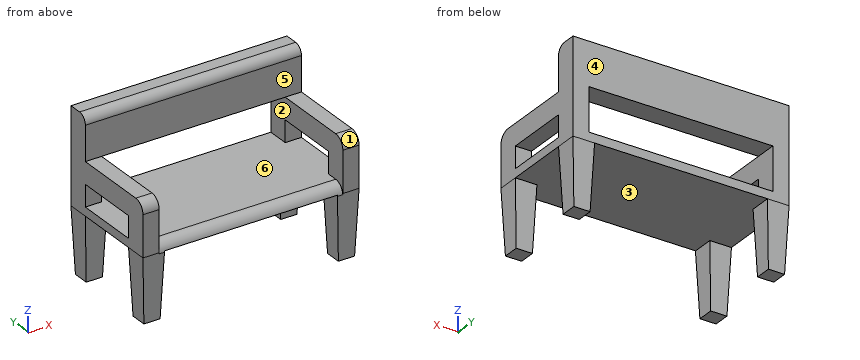
```python
from build123d import *

# Parameters (mm, degrees)
F0_W         = 200
F0_H         = 100
F1_DEPTH     = 8
F2_W         = 20
F2_H         = 20
F4_W         = 15
F4_H         = 15
F8_W         = 15
F8_H         = 20
F9_DEPTH     = 80
F11_W        = 20
F11_H        = 40
F12_DEPTH    = 170
F14_DEPTH    = 80
F15_W        = 15
F15_H        = 20
F16_DEPTH    = 20
F18_R        = 10
F19_R        = 10
F20_T1_DEPTH = 170
F21_R        = 8


# Not quite as in the source:
# - a fillet or chamfer that OpenCascade refuses, or shapes differently, is made with other operations: its cross-section is extruded or revolved along the edge and cut away or added


with BuildPart() as f1:
    # F0 (on Top) → F1 (new body)
    with BuildSketch(Plane.XY):
        Rectangle(F0_W, F0_H)
    extrude(amount=F1_DEPTH)

    # F2 (on face) → F5 section 0
    with BuildSketch(Plane(origin=(0, 0, 0), x_dir=(1, 0, 0), z_dir=(0, 0, -1))):
        with Locations((-90, 40)):
            Rectangle(F2_W, F2_H)
    # F4 (on offset) → F5 section 1
    with BuildSketch(Plane.XY.offset(-60)):
        with Locations((-90, -40)):
            Rectangle(F4_W, F4_H)
    loft()

    # F6: F1 across plane


with BuildPart() as f1_1:
    add(f1.part)
    add(f1.part.mirror(Plane.XZ))

    # F7: F1 across plane


with BuildPart() as f1_2:
    add(f1_1.part)
    add(f1_1.part.mirror(Plane.YZ))

    # F8 (on face) → F9 (join)
    with BuildSketch(Plane.XY.offset(8)):
        with Locations((-92.5, 40)):
            Rectangle(F8_W, F8_H)
    extrude(amount=F9_DEPTH)

    # F10: F1 across plane


with BuildPart() as f1_3:
    add(f1_2.part)
    add(f1_2.part.mirror(Plane.YZ))

    # F11 (on face) → F12 (join)
    with BuildSketch(Plane.YZ.offset(-85)):
        with Locations((40, 68)):
            Rectangle(F11_W, F11_H)
    extrude(amount=F12_DEPTH)

    # F13 (on face) → F14 (join)
    with BuildSketch(Plane.XZ.offset(-30)):
        Polygon((-85, 28), (-85, 48), (-92.5, 48), (-100, 48), (-100, 28), align=None)
    extrude(amount=F14_DEPTH)

    # F15 (on face) → F16 (join)
    with BuildSketch(Plane(origin=(0, 0, 28), x_dir=(1, 0, 0), z_dir=(0, 0, -1))):
        with Locations((-92.5, 40)):
            Rectangle(F15_W, F15_H)
    extrude(amount=F16_DEPTH)

    # F17: F1 across plane


with BuildPart() as f1_4:
    add(f1_3.part)
    add(f1_3.part.mirror(Plane.YZ))

    # F18
    f18_edges = [f1_4.edges().sort_by_distance(p)[0] for p in [
        (92.5, -50, 48),
    ]]
    fillet(f18_edges, radius=F18_R)

    # F19
    f19_edges = [f1_4.edges().sort_by_distance(p)[0] for p in [
        (-92.5, -50, 48),
    ]]
    fillet(f19_edges, radius=F19_R)

    # F20: fillet of radius 10 on 1 edges, made by hand

    # F20_s2 → F20_t1 (cut)
    with BuildSketch(Plane.YZ.offset(-85)):
        with BuildLine():
            ThreePointArc((-50, -2), (-47.0710678119, 5.0710678119), (-40, 8))
            Line((-40, 8), (-50, 8))
            Line((-50, 8), (-50, -2))
        make_face()
    extrude(amount=F20_T1_DEPTH, mode=Mode.SUBTRACT)

    # F21
    f21_edges = [f1_4.edges().sort_by_distance(p)[0] for p in [
        (0, 30, 88),
    ]]
    fillet(f21_edges, radius=F21_R)


solid = f1_4.part
```
For this review, take the finished solid that the model builds, in its own axes (mm). Face numbers are marked on the shaded views. A direction names the side the tool comes from. Give positions to 0.01 mm unless a question says otherwise; leave off trailing zeros. Write each loop counter-clockwise with the first axis right and the second up, starting at its lowest first coordinate (ties: lowest second). Pieces come first, ordered by that corner, then holes.
Item 1: The part is to be moulded in two halves that separate along Y. For the marked faces 1, 2 and 3, say which applies: +Y half, -Y half, draft (parallel to the pull), parting line (faces both ways), or undercut.
Item 2: Take a section at D-D (z = 52.5). Give the boundary of the cut face in (x, y), and give its area (3 significant figures).
Item 3: Insertion check: P1, Ø16, axis at x = 34, y = 42.5, coming from the -Z side; P2, Ø7.5, axis at x = 89.5, y = 12, coming from the +Z side; P3, Ø12, axis at x = 30.5, y = -17.5, coming from the +Z side. Each pin has a flat end and moves straight along its axis. Give the tip position at first contact, or say it passes through.
Item 4: Machinability: for the marked faces 4, 5 and 6, which of the approach directions +Z, -Z, +X, -X, +Y, -Y give a long, thin tool a straight path to every point of the face, cutting with its end or side? Answer none if there is none.
Item 5: Take a section at A-A (y = 12). Give the boundary of the cut face in (x, z), and give its area (3 significant figures).
Item 6: Take a section at C-C (z = 11.5). Give the boundary of the cut face in (x, y), and give its area (3 significant figures).
Item 7: Take a section at B-B (x = 76). Give the boundary of the cut face in (y, z), and give its area (3 significant figures).
Item 8: Wall thickness on probe 1 along Z at (x, y) = (-40, 43.5); probe 2 along X at (y, z) = (3.5, 40.5); probe 3 along Z at (x, y) = (-62, -13): over which ranges is each line inside the solid? List them lowest first.
Established:
1. face 1: -Y half
1. face 2: draft
1. face 3: undercut
2. outline: (-100, 30) - (100, 30) - (100, 50) - (-100, 50) - close
2. area: 4,000 mm2
3. P1: stops at z = 0
3. P2: stops at z = 48
3. P3: stops at z = 8
4. face 4: +Z, -Z, +X, -X, +Y
4. face 5: +Z, +X, -X, -Y
4. face 6: none
5. outline: (-100, 0) - (100, 0) - (100, 8) - (-100, 8) - close; (-100, 28) - (-85, 28) - (-85, 48) - (-100, 48) - close; (85, 28) - (100, 28) - (100, 48) - (85, 48) - close
5. area: 2,200 mm2
6. outline: (-100, -50) - (-85, -50) - (-85, -30) - (-100, -30) - close; (-100, 30) - (-85, 30) - (-85, 50) - (-100, 50) - close; (85, -50) - (100, -50) - (100, -30) - (85, -30) - close; (85, 30) - (100, 30) - (100, 50) - (85, 50) - close
6. area: 1,200 mm2
7. outline: (-49.8, 0) - (50, 0) - (50, 8) - (-40, 8) arc R10 ccw to start; (30, 48) - (50, 48) - (50, 88) - (38, 88) arc R8 ccw to (30, 80) - close
7. area: 1,560 mm2
8. probe 1: z = 0 to 8, 48 to 88
8. probe 2: x = -100 to -85, 85 to 100
8. probe 3: z = 0 to 8
